Build history of the part. All positions in model axes, mm. A direction names the side the tool comes from. Round coordinates to 2 decimals unless told otherwise and drop trailing zeros. Loops run counter-clockwise (first coordinate to the right, second up) from the corner with the lowest first, then second, coordinate; pieces in that order, holes last. Notation, with made-up numbers: (13.25, -34) - (53.25, -34) arc R23 ccw to (53.25, -4) - close; hole circle Ø4 at (72, 24.25). An arc over 180 degrees is marked (long way). Put each result on its own line as item: value. Start each with the question number.
from build123d import *

# Parameters (mm, degrees)
F0_R          = 29.3309291426
F1_DEPTH      = 84.836
F2_T          = -7.62
F3_R          = 6.1041032484
F4_DEPTH      = 29.3319291426
F4_DEPTH_BACK = 29.3319291426


with BuildPart() as f1:
    # F0 (on Top) → F1 (new body)
    with BuildSketch(Plane.XY):
        Circle(F0_R)
    extrude(amount=F1_DEPTH)

    # F2
    f2_openings = [f1.faces().sort_by_distance(p)[0] for p in [
        (0, 0, 0),
    ]]
    offset(amount=F2_T, openings=f2_openings)

    # F3 (on Front) → F4 (cut, two sides)
    with BuildSketch(Plane.XZ) as f4_sk:
        with Locations((0, 51.1526353657)):
            Circle(F3_R)
    extrude(amount=-F4_DEPTH, mode=Mode.SUBTRACT)
    extrude(f4_sk.sketch, amount=F4_DEPTH_BACK, mode=Mode.SUBTRACT)


solid = f1.part
1) Slice it at D-D, the plane y = -24. Write the cut outline in (x, z), and give its area (3 significant figures).
2) Which spindle directions (+Z, -Z, +X, -X, +Y, -Y) get a long thin tool onto all of the face, cutting with end or side? Do faces 1 (the face through (0, 0, 84.836)), 2 (the face through (-4.707, -21.195, 38.067)). Say none if no direction does.
3) Slice it at A-A, the plane x = 0. Write the cut outline in (y, z).
4) Drill centre lines: line 1 (Z direction, x = 0, y = -23); line 2 (Y direction, x = 0.5, z = 77.5); line 3 (Y direction, x = 0, z = 32). Where is each one in solid material? Low to high. Write a range as [from, to].
5) Slice it at C-C, the plane y = -6.5. Write the cut outline in (x, z), and give its area (3 significant figures).
6) Drop flat-ended pins along their axis: pin 1 Ø2 at (y, z) = (0.5, 10) entering from -X; pin 2 Ø3 at (x, z) = (16, 71) entering from +Y; pin 3 Ø4 at (x, z) = (4, 32) entering from -Y; pin 4 Ø1 at (x, y) = (22, 23) entering from -Z. Give the stop position or say it passes through.
7) Pull direction X, two halves, no side cores. Call faces 3 (the face through (-4.844, -25.021, 47.438)), 4 (the face through (-6.358, -28.633, 41.824)), 5 (the face through (0, 22, 0)): pulls with the +X half, pulls with the -X half, needs draft (parallel to the pull), parting line crosses it, or undercut.
8) Slice it at B-B, the plane z = 47. Write the cut outline in (x, y).
Taken from the geometry:
1. outline: (-16.86, 0) - (16.86, 0) - (16.86, 84.84) - (-16.86, 84.84) - close; hole circle Ø12.21 at (0, 51.15)
1. area: 2,740 mm2
2. face 1: +Z, +X, -X, +Y, -Y
2. face 2: -Z
3. outline: (-29.33, 0) - (-21.71, 0) - (-21.71, 45.05) - (-29.33, 45.05) - close; (-29.33, 57.26) - (-21.71, 57.26) - (-21.71, 77.22) - (21.71, 77.22) - (21.71, 57.26) - (29.33, 57.26) - (29.33, 84.84) - (-29.33, 84.84) - close; (21.71, 0) - (29.33, 0) - (29.33, 45.05) - (21.71, 45.05) - close
4. line 1: z = [0, 45.05], [57.26, 84.84]
4. line 2: y = [-29.33, 29.33]
4. line 3: y = [-29.33, -21.71], [21.71, 29.33]
5. outline: (-28.6, 0) - (-20.72, 0) - (-20.72, 77.22) - (20.72, 77.22) - (20.72, 0) - (28.6, 0) - (28.6, 84.84) - (-28.6, 84.84) - close
5. area: 1,650 mm2
6. pin 1: stops at x = -29.33
6. pin 2: stops at y = 25.5
6. pin 3: stops at y = -29.26
6. pin 4: passes through
7. face 3: undercut
7. face 4: parting line crosses it
7. face 5: needs draft
8. outline: (-4.47, -28.99) - (-4.47, -21.24) arc R21.71 cw to (-4.47, 21.24) - (-4.47, 28.99) arc R29.33 ccw to start; (4.47, -28.99) arc R29.33 ccw to (4.47, 28.99) - (4.47, 21.24) arc R21.71 cw to (4.47, -21.24) - close
